Part model, mm, in its own coordinate system. Coordinates: 2 decimals unless noted, no trailing zeros.
1) Wall check: L1, parallel to Y at x = 2.5, z = 0; L2, parallel to Z at x = 0.5, y = -10. Give the ranges that are in metal, low to high.
2) Pin check, flat tips, straight feed: pin 1 Ø1 at (x, y) = (2.5, 74) entering from -Z; pin 2 Ø1.5 at (x, z) = (3.5, -33) entering from -Y; pin 3 Ø1.5 at (x, z) = (3.5, -69.5) entering from -Y. Stop position of each tip, or through.
3) Cut at A-A (z = 0). Give the number of separate pieces and of enclosed holes in the cut face, and give its area (3 significant figures).
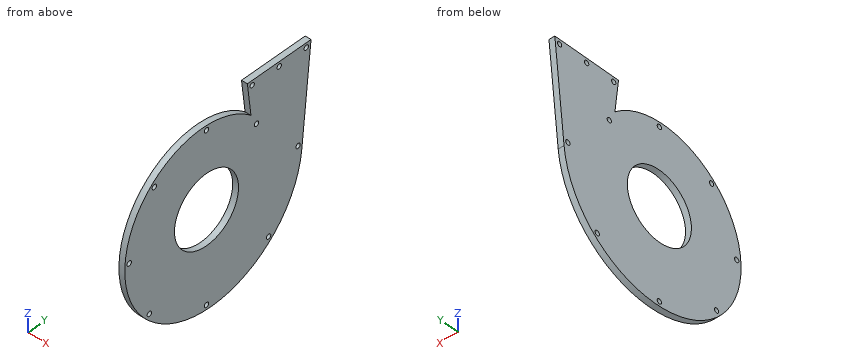
```python
from build123d import *

# Parameters (mm, degrees)
BOSS_EXTRUDE1_DEPTH = 6.35
SKETCH11_R          = 2.55
CUT_EXTRUDE1_DEPTH  = 7.3500001
SKETCH12_R          = 37.5
CUT_EXTRUDE3_DEPTH  = 7.3500001


with BuildPart() as part:
    # Sketch10 → Boss-Extrude1 (new body)
    with BuildSketch(Plane(origin=(0, 0, 0), x_dir=(0, 0, -1), z_dir=(1, 0, 0))):
        with BuildLine():
            Line((-65.56933734, 52.009531221), (-100.935679824, 47.808985699))
            Line((-100.935679824, 47.808985699), (-100.935679824, 122.29075479))
            Line((-100.935679824, 122.29075479), (5.970340966, 111.513169224))
            add(Edge.make_bspline(
                [(5.970340966, 111.513169224), (9.050174513, 111.20267998), (15.195754527, 110.322198965), (27.224457069, 107.560584888), (41.672600889, 102.269141777), (57.583217011, 93.200335773), (76.34944741, 77.877389952), (94.274449289, 53.53377411), (104.843460982, 19.443777188), (103.677945005, -15.636484697), (91.289552438, -47.848309946), (69.405777179, -73.770277552), (40.739036605, -90.784845908), (8.654881454, -97.341351398), (-23.220610692, -93.091773694), (-51.414586087, -78.887047742), (-72.979776783, -56.641213756), (-85.804607758, -29.085280645), (-88.816261681, 0.571051967), (-83.191535024, 24.252063706), (-74.366432128, 41.075630131), (-68.698633198, 48.535069634), (-65.56933734, 52.009531221)],
                knots=[0.103071112, 0.103071112, 0.103071112, 0.103071112, 0.117085626, 0.13110014, 0.159129168, 0.187158196, 0.215187223, 0.271245279, 0.327303334, 0.38336139, 0.439419445, 0.495477501, 0.551535556, 0.607593612, 0.663651667, 0.719709723, 0.775767778, 0.831825834, 0.887883889, 0.943941945, 0.971970972, 1, 1, 1, 1], degree=3))
        make_face()
    extrude(amount=BOSS_EXTRUDE1_DEPTH)

    # Sketch11 → Cut-Extrude1 (cut, through all)
    with BuildSketch(Plane(origin=(6.35, 0, 0), x_dir=(0, 0, -1), z_dir=(1, 0, 0))):
        with Locations((-95.935679824, 116.761342324)):
            Circle(SKETCH11_R)
        with Locations((-95.935679824, 53.437991421)):
            Circle(SKETCH11_R)
        with Locations((-95.935679824, 85.099666873)):
            Circle(SKETCH11_R)
        with Locations((-52.956120261, 58.54277704)):
            Circle(SKETCH11_R)
        with Locations((0, -90.448962865)):
            Circle(SKETCH11_R)
        with Locations((-82.20247918, 0)):
            Circle(SKETCH11_R)
        with Locations((98.695882227, 0)):
            Circle(SKETCH11_R)
        with Locations((0, 107.089716811)):
            Circle(SKETCH11_R)
        with Locations((-61.03999449, -61.03999449)):
            Circle(SKETCH11_R)
        with Locations((66.874078846, -66.874078846)):
            Circle(SKETCH11_R)
        with Locations((72.70516699, 72.70516699)):
            Circle(SKETCH11_R)
    extrude(amount=-CUT_EXTRUDE1_DEPTH, mode=Mode.SUBTRACT)

    # Sketch12 → Cut-Extrude3 (cut, through all)
    with BuildSketch(Plane(origin=(0, 0, 0), x_dir=(0, 0, -1), z_dir=(1, 0, 0))):
        Circle(SKETCH12_R)
    extrude(amount=CUT_EXTRUDE3_DEPTH, mode=Mode.SUBTRACT)


solid = part.part
```
Geometry check:
1. L1: y = -95.46 to -93, -87.9 to -37.5, 37.5 to 104.54, 109.64 to 112.12
1. L2: z = -102.71 to -36.14, 36.14 to 87.24
2. pin 1: stops at z = -78.65
2. pin 2: stops at y = -91.73
2. pin 3: stops at y = -71.88
3. separate pieces: 4
3. enclosed holes: 0
3. area: 777 mm2
